Here's how the part is built. I have some questions about the finished solid (model axes, mm). A direction names the side the tool comes from. Coordinates: 2 decimals unless noted, no trailing zeros. Write each loop counter-clockwise with the first axis right and the second up, starting at its lowest first coordinate (ties: lowest second). Pieces come first, ordered by that corner, then holes.
Item 1: I want a section at B-B (x = 0). Please give me the cut outline in (y, z).
Item 2: I want a section at D-D (x = 7). Please give me the cut outline in (y, z), and give its area (3 significant figures).
Item 3: Please list where these lines run through material, in increasing order: line 1 (Y direction, x = -5.75, z = 0); line 2 (Z direction, x = 0, y = 10.5); line 3 (Z direction, x = 0.5, y = 12.5).
Item 4: I want a section at A-A (z = 0). Please give me the cut outline in (x, y), and give its area (4 significant figures).
Item 5: For faces 4 (the face through (2, 15, 6)), 5 (the face through (1.84, 8.11, 1.69)), 6 (the face through (-5, 4.3, 1.5)), which set-ups out of +Z, -Z, +X, -X, +Y, -Y let a thin tool reach every point of the face, with its end or its side?
Item 6: I want a section at C-C (y = 15.25). Please give me the cut outline in (x, z).
Item 7: If we mould it in two halves opening along X, with no side actions, what happens to faces 1 (the face through (-1.5, 4.3, -5)), 2 (the face through (1.73, 15.49, -7.81)), 3 (the face through (-2, 16, -2))? For each: pulls with the +X half, pulls with the -X half, needs draft (parallel to the pull), parting line crosses it, or undercut.
Item 8: I'm going to push flat-ended pins straight in: P1, Ø3, axis at x = 2, z = 1.5, coming from the -Y side; P2, Ø4, axis at x = 5.5, y = 3, coming from the -Z side; P3, Ø4.5, axis at x = 0, z = 0, coming from the +Y side; P4, Ø3, axis at y = 7.5, z = 5.5, coming from the +X side. Where does each tip first touch, or does it pass through?
from build123d import *

# Parameters (mm, degrees)
ESQUISSE2_R             = 1.5
ENL_V_MAT_EXTRU_1_DEPTH = 9
ESQUISSE3_R             = 1.5
ENL_V_MAT_EXTRU_2_DEPTH = 9.0000001


with BuildPart() as part:
    # Esquisse1 → Révolution1 (revolve)
    with BuildSketch(Plane.XY):
        Polygon((-2.5, 0), (-2.5, 16), (-8, 16), (-8, 15), (-6, 15), (-6, 8.5), (-8, 8.5), (-8, 0), align=None)
    revolve(axis=Axis((0, 0, 0), (0, 1, 0)))

    # Esquisse2 → Enlèv. mat.-Extru.1 (cut, through all)
    with BuildSketch(Plane(origin=(0, 0, 0), x_dir=(0, 0, -1), z_dir=(1, 0, 0))):
        with Locations((0, 4.25)):
            Circle(ESQUISSE2_R)
    extrude(amount=-ENL_V_MAT_EXTRU_1_DEPTH, mode=Mode.SUBTRACT)

    # Esquisse3 → Enlèv. mat.-Extru.2 (cut, through all)
    with BuildSketch(Plane.XY):
        with Locations((0, 4.25)):
            Circle(ESQUISSE3_R)
    extrude(amount=-ENL_V_MAT_EXTRU_2_DEPTH, mode=Mode.SUBTRACT)


solid = part.part
Answer:
1. outline: (0, -8) - (2.75, -8) - (2.75, -2.5) - (0, -2.5) - close; (0, 2.5) - (16, 2.5) - (16, 8) - (15, 8) - (15, 6) - (8.5, 6) - (8.5, 8) - (0, 8) - close; (5.75, -8) - (8.5, -8) - (8.5, -6) - (15, -6) - (15, -8) - (16, -8) - (16, -2.5) - (5.75, -2.5) - close
2. outline: (0, -3.87) - (8.5, -3.87) - (8.5, 3.87) - (0, 3.87) - close; (15, -3.87) - (16, -3.87) - (16, 3.87) - (15, 3.87) - close
2. area: 73.6 mm2
3. line 1: y = 0 to 2.75, 5.75 to 16
3. line 2: z = -6 to -2.5, 2.5 to 6
3. line 3: z = -5.98 to -2.45, 2.45 to 5.98
4. outline: (-8, 0) - (-2.5, 0) - (-2.5, 2.75) - (-8, 2.75) - close; (-8, 5.75) - (-2.5, 5.75) - (-2.5, 16) - (-8, 16) - (-8, 15) - (-6, 15) - (-6, 8.5) - (-8, 8.5) - close; (2.5, 0) - (8, 0) - (8, 8.5) - (6, 8.5) - (6, 15) - (8, 15) - (8, 16) - (2.5, 16) - close
4. area: 133.5 mm2
5. face 4: none
5. face 5: +Y, -Y
5. face 6: -X
6. outline: circle Ø16 at (0, 0); hole circle Ø5 at (0, 0)
7. face 1: undercut
7. face 2: parting line crosses it
7. face 3: needs draft
8. P1: stops at y = 0
8. P2: stops at z = -7.19
8. P3: passes through
8. P4: stops at x = 6.93
